Check sheet for the modelled part. Datum: model origin and axes. Units: mm. A direction names the side the tool comes from. Round coordinates to 2 decimals unless told otherwise and drop trailing zeros. Loops run counter-clockwise (first coordinate to the right, second up) from the corner with the lowest first, then second, coordinate; pieces in that order, holes last. Notation, with made-up numbers: (68.25, -39) - (126.25, -39) arc R27 ccw to (126.25, -3) - close; hole circle Ø5 at (-36, 36.25). An arc over 180 degrees is marked (long way). Return JSON: item names as keys, results as strings.
from build123d import *

# Parameters (mm, degrees)
SKETCH_1_W          = 170
SKETCH_1_H          = 40
SKETCH_1_R          = 1.6
EXTRUDE_1_DEPTH     = 3
SKETCH_2_R          = 1.6
CUT_EXTRUDE_1_DEPTH = 4
SKETCH_3_W          = 15
SKETCH_3_H          = 6
EXTRUDE_2_DEPTH     = 6


with BuildPart() as part:
    # 草图1 → 凸台-拉伸1 (new body)
    with BuildSketch(Plane.XY):
        with Locations((-6.503957784, -3.970976253)):
            Rectangle(SKETCH_1_W, SKETCH_1_H)
        with Locations((-71.503957784, 8.529023747)):
            Circle(SKETCH_1_R, mode=Mode.SUBTRACT)
        with Locations((-59.003957784, -3.970976253)):
            Circle(SKETCH_1_R, mode=Mode.SUBTRACT)
        with Locations((-71.503957784, -16.470976253)):
            Circle(SKETCH_1_R, mode=Mode.SUBTRACT)
        with Locations((-84.003957784, -3.970976253)):
            Circle(SKETCH_1_R, mode=Mode.SUBTRACT)
        with Locations((70.996042216, -3.970976253)):
            Circle(SKETCH_1_R, mode=Mode.SUBTRACT)
        with Locations((58.496042216, 8.529023747)):
            Circle(SKETCH_1_R, mode=Mode.SUBTRACT)
        with Locations((58.496042216, -16.470976253)):
            Circle(SKETCH_1_R, mode=Mode.SUBTRACT)
        with Locations((45.996042216, -3.970976253)):
            Circle(SKETCH_1_R, mode=Mode.SUBTRACT)
    extrude(amount=EXTRUDE_1_DEPTH)

    # 草图2 → 切除-拉伸1 (cut, through all)
    with BuildSketch(Plane(origin=(0, 0, 0), x_dir=(-1, 0, 0), z_dir=(0, 0, -1))):
        with Locations((-36.496042216, 12.029023747)):
            Circle(SKETCH_2_R)
        with Locations((-36.496042216, -19.970976253)):
            Circle(SKETCH_2_R)
        with Locations((49.503957784, 12.029023747)):
            Circle(SKETCH_2_R)
        with Locations((49.503957784, -19.970976253)):
            Circle(SKETCH_2_R)
    extrude(amount=-CUT_EXTRUDE_1_DEPTH, mode=Mode.SUBTRACT)

    # 草图3 → 凸台-拉伸2 (add)
    with BuildSketch(Plane(origin=(0, 0, 0), x_dir=(-1, 0, 0), z_dir=(0, 0, -1))):
        with Locations((-70.996042216, 13.029023747)):
            Rectangle(SKETCH_3_W, SKETCH_3_H)
        with Locations((-70.996042216, -20.970976253)):
            Rectangle(SKETCH_3_W, SKETCH_3_H)
        with Locations((84.003957784, 13.029023747)):
            Rectangle(SKETCH_3_W, SKETCH_3_H)
        with Locations((84.003957784, -20.970976253)):
            Rectangle(SKETCH_3_W, SKETCH_3_H)
    extrude(amount=EXTRUDE_2_DEPTH)


solid = part.part
Q1. Depth check by flat-ended pin: P1, Ø3.5, axis at x = -49.5, y = 12.03, coming from the -Z side; P2, Ø4, axis at x = 46, y = -3.97, coming from the +Z side. Enter the tip coordinate at first touch or a pass-through.
Answer key:
{"P1": "stops at z = 0", "P2": "stops at z = 3"}
Q2. Tool access check on faces 1 (the face through (-69.98, -15.99, 1.48)), 2 (the face through (71, 10.029, -3)), 3 (the face through (63.496, -21, -3)). Record the directions out of +Z, -Z, +X, -X, +Y, -Y that give a thin tool (end or side, any length) a straight path to the whole face; none if there is none.
Answer key:
{"face 1": "+Z, -Z", "face 2": "-Z, +X, -X", "face 3": "-Z, +Y, -Y"}
Q3. Sectioned sample at B-B (x = -45.5). Enter the section's corners in (y, z).
Answer key:
{"outline": "(-23.97, 0) - (16.03, 0) - (16.03, 3) - (-23.97, 3) - close"}
Q4. Sectioned sample at A-A (z = -1.75). Enter the section's corners in (x, y).
Answer key:
{"outline": "(-91.5, -23.97) - (-76.5, -23.97) - (-76.5, -17.97) - (-91.5, -17.97) - close; (-91.5, 10.03) - (-76.5, 10.03) - (-76.5, 16.03) - (-91.5, 16.03) - close; (63.5, -23.97) - (78.5, -23.97) - (78.5, -17.97) - (63.5, -17.97) - close; (63.5, 10.03) - (78.5, 10.03) - (78.5, 16.03) - (63.5, 16.03) - close"}
Q5. Draft check along X on faces 4 (the face through (78.496, -4, 1)), 5 (the face through (-76.504, -21, -3)), 6 (the face through (-91.504, -4.3, 0.4)), 7 (the face through (71, -21, -6)). Enter one of: released by +X, released by -X, zero draft, split by the parting line, or undercut.
Answer key:
{"face 4": "released by +X", "face 5": "undercut", "face 6": "released by -X", "face 7": "zero draft"}
Q6. Sectioned sample at C-C (y = 1). Enter the section's corners in (x, z), plus the area to 3 significant figures.
Answer key:
{"outline": "(-91.5, 0) - (78.5, 0) - (78.5, 3) - (-91.5, 3) - close", "area": "510 mm²"}
Q7. Scan lines: probe 1 along Y at (x, z) = (68, -4.75); probe 2 along Z at (x, y) = (69, -6); probe 3 along X at (y, z) = (10.5, -1.5). Record each from-to range of solid material in increasing order. Write a range as [from, to].
Answer key:
{"probe 1": "y = [-23.97, -17.97], [10.03, 16.03]", "probe 2": "z = [0, 3]", "probe 3": "x = [-91.5, -76.5], [63.5, 78.5]"}
